Geometry: final body of the model. Coordinates: model frame, mm. Face numbers are marked on the shaded views. A direction names the side the tool comes from. Give positions to 0.01 mm unless a question says otherwise; leave off trailing zeros. Write each loop counter-clockwise with the first axis right and the second up, starting at its lowest first coordinate (ties: lowest second). Pieces come first, ordered by that corner, then holes. Notation, with made-up numbers: M -13.75,67 L 8.25,67 A11 cw 8.25,84 Z; hole C 19,80.5 d1. An arc over 180 degrees is marked long. Answer as a JSON object with one key per item and string values.
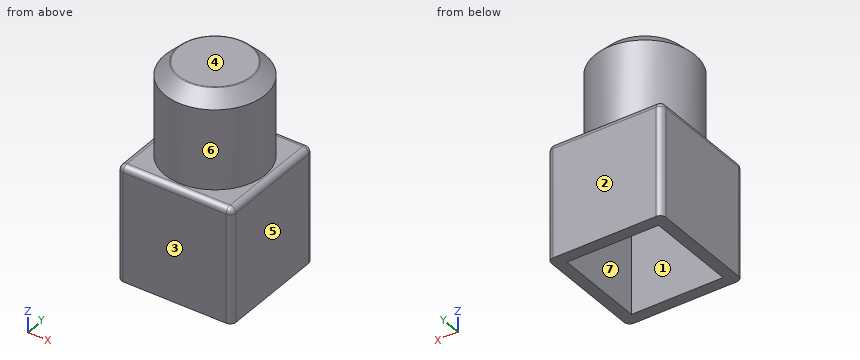
from build123d import *

# Parameters (mm, degrees)
F0_W     = 25.4
F0_H     = 25.4
F1_DEPTH = 12.7
F2_R     = 11.1125
F3_DEPTH = 20.6375
F4_SIZE  = 2.9718
F5_R     = 0.254
F6_R     = 1.27
F7_R     = 1.27
F8_R     = 1.27
F9_R     = 1.27
F10_T    = -2.54


with BuildPart() as f1:
    # F0 (on Front) → F1 (new body, symmetric)
    with BuildSketch(Plane.XZ):
        Rectangle(F0_W, F0_H)
    extrude(amount=F1_DEPTH, both=True)

    # F2 (on face) → F3 (join)
    with BuildSketch(Plane.XY.offset(12.7)):
        Circle(F2_R)
    extrude(amount=F3_DEPTH)

    # F4
    f4_edges = [f1.edges().sort_by_distance(p)[0] for p in [
        (-11.1125, 0, 33.3375),
    ]]
    chamfer(f4_edges, length=F4_SIZE)

    # F5
    f5_edges = [f1.edges().sort_by_distance(p)[0] for p in [
        (-8.1407, 0, 33.3375),
    ]]
    fillet(f5_edges, radius=F5_R)

    # F6
    f6_edges = [f1.edges().sort_by_distance(p)[0] for p in [
        (0, -12.7, 12.7),
    ]]
    fillet(f6_edges, radius=F6_R)

    # F7
    f7_edges = [f1.edges().sort_by_distance(p)[0] for p in [
        (12.7, 0.635, 12.7),
    ]]
    fillet(f7_edges, radius=F7_R)

    # F8
    f8_edges = [f1.edges().sort_by_distance(p)[0] for p in [
        (-12.7, 0.635, 12.7),
    ]]
    fillet(f8_edges, radius=F8_R)

    # F9
    f9_edges = [f1.edges().sort_by_distance(p)[0] for p in [
        (0, 12.7, 12.7),
    ]]
    fillet(f9_edges, radius=F9_R)

    # F10
    f10_openings = [f1.faces().sort_by_distance(p)[0] for p in [
        (0, 0, -12.7),
    ]]
    offset(amount=F10_T, openings=f10_openings, kind=Kind.INTERSECTION)


solid = f1.part
1) Pull-direction query (Y, two-part tool) for the marked faces 1, 2, 3 and 4; classes: pulls with the +Y half, pulls with the -Y half, needs draft (parallel to the pull), parting line crosses it, or undercut.
Geometry check:
{"face 1": "undercut", "face 2": "pulls with the +Y half", "face 3": "pulls with the -Y half", "face 4": "needs draft"}
2) Contact query for flat-ended pins moving along their axis: P1, Ø2, axis at x = 9.5, z = 13.5, coming from the +Y side; P2, Ø1.5, axis at x = 10, z = 14.5, coming from the +Y side; P3, Ø12, axis at y = 5, z = 18.5, coming from the +X side. Output: stop coordinate, or through.
Geometry check:
{"P1": "stops at y = 12.11", "P2": "stops at y = 6.16", "P3": "stops at x = 12.11"}
3) Line query: line 1 (Y direction, x = 9, z = -7.5); line 2 (Y direction, x = 0, z = 20.5). Output: solid intervals per line, ascending. Write a range as from..to.
Geometry check:
{"line 1": "y = -12.7..-10.16, 10.16..12.7", "line 2": "y = -11.11..-8.57, 8.57..11.11"}
4) Set-up query: the marked faces 5, 6 and 7. Return all of +Z, -Z, +X, -X, +Y, -Y with unobstructed straight access to the full face (end or side cutting, diameter ignored); none if empty.
Geometry check:
{"face 5": "+Z, -Z, +X, +Y, -Y", "face 6": "+Z", "face 7": "-Z"}
5) Cut plane A-A on z = 5. Return loops of the section in (x, y).
Geometry check:
{"outline": "M -12.7,-11.43 A1.27 ccw -11.43,-12.7 L 11.43,-12.7 A1.27 ccw 12.7,-11.43 L 12.7,11.43 A1.27 ccw 11.43,12.7 L -11.43,12.7 A1.27 ccw -12.7,11.43 Z; hole M -10.16,-10.16 L 10.16,-10.16 L 10.16,10.16 L -10.16,10.16 Z"}
6) Cut plane D-D on z = 14. Return loops of the section in (x, y) (1 decimal), and give its area (3 significant figures).
Geometry check:
{"outline": "C 0,0 d22.2; hole C 0,0 d17.1", "area": "157 mm2"}
7) Cut plane B-B on y = 0. Return loops of the section in (x, z).
Geometry check:
{"outline": "M -12.7,-12.7 L -10.16,-12.7 L -10.16,10.16 L -8.57,10.16 L -8.57,29.31 L -7.09,30.8 L 7.09,30.8 L 8.57,29.31 L 8.57,10.16 L 10.16,10.16 L 10.16,-12.7 L 12.7,-12.7 L 12.7,11.43 A1.27 ccw 11.43,12.7 L 11.11,12.7 L 11.11,30.37 L 8.22,33.26 A0.25 ccw 8.04,33.34 L -8.04,33.34 A0.25 ccw -8.22,33.26 L -11.11,30.37 L -11.11,12.7 L -11.43,12.7 A1.27 ccw -12.7,11.43 Z"}
